Autodesk Inventor part; units mm, degrees
ref_plane "YZ Plane" through (0, 0, 0) normal (1, 0, 0) x (0, 1, 0)
ref_plane "XZ Plane" through (0, 0, 0) normal (0, 1, 0) x (-1, 0, 0)
ref_plane "XY Plane" through (0, 0, 0) normal (0, 0, 1) x (1, 0, 0)
sketch "Sketch3" plane through (0, 0, 0) normal (0, 1, 0) x (-1, 0, 0)
  line L0 (-11.3909, 27.5) -> (11.3909, 27.5)
  line L1 (11.3909, 27.5) -> (27.5, 11.3909)
  line L2 (27.5, 11.3909) -> (27.5, -11.3909)
  line L3 (27.5, -11.3909) -> (11.3909, -27.5)
  line L4 (11.3909, -27.5) -> (-11.3909, -27.5)
  line L5 (-11.3909, -27.5) -> (-27.5, -11.3909)
  line L6 (-27.5, -11.3909) -> (-27.5, 11.3909)
  line L7 (-27.5, 11.3909) -> (-11.3909, 27.5)
  circle A0 centre (0, 0) radius 29.7658
  circle A1 centre (0, 0) radius 27.5
  circle A2 centre (0, 0) radius 21
  circle A3 centre (0, 0) radius 31.7658
  line L8 (0, 0) -> (-27.5, 0)
  line L9 (-27.5, 0) -> (-27.5, 83)
  line L10 (-27.5, 83) -> (0, 83)
  line L11 (0, 83) -> (0, 0)
  line L12 (0, 83) -> (-7.5939, 83)
  line L13 (-7.5939, 83) -> (-7.5939, 166)
  line L14 (-7.5939, 166) -> (0, 166)
  line L15 (0, 166) -> (0, 83)
  line L16 (0, 166) -> (-47, 166)
  line L17 (-47, 166) -> (-47, 171)
  line L18 (-47, 171) -> (0, 171)
  line L19 (0, 171) -> (0, 166)
  circle A4 centre (-47, 168.5) radius 7.5939
  dimension "oSW" = 55
  dimension "oIntDia" = 42
  dimension "d16" = 2
  dimension "oWheelDia" = 94
  dimension "d51" = 5
  dimension "d52" = 15.1878
  dimension "oStemHeight" = 171
  dimension "d57" = 15.1878
  dimension "d58" = 22.7817
revolve "Revolution1" add sketch "Sketch3" angle 360 about axis through (0, 0, 166) along (0, 0, -1) picked at (-6.365, 27.9172) picked at (-16.0373, 26.4927) picked at (-1.7883, 25.1572) picked at (-13.8245, 1.5576) contours A0 L11 L0 | L0 A1 L7 | L7 A0 | A0 L9 A3 L11 | L11 A2 L8 A1 | A1 L6 L7 | L11 L8 A2 | L9 L10 L11 A3 | L10 L13 L14 L15 | L14 L16 A4 L18 L19 | A4 L18 L17 L16 | L16 L17 L18 A4
extrude "Extrusion1" add sketch "Sketch3" along normal mid plane 82 separate body contours L0 A1 L7 | L0 L1 A1 | L11 A2 L8 A1 | A1 L8 A2 L11 | A1 L6 L7 | L1 L2 A1 | A1 L5 L6 | L2 L3 A1 | A1 L4 L5 | L3 L4 A1
extrude "Extrusion12" cut sketch "Sketch3" along normal through all both and the other way through all contours L11 L8 A2 | A2 L8 L11
extrude "Extrusion2" add sketch "Sketch3" along normal mid plane 60 contours A0 L11 L0 | L7 A0 | A0 L9 A3 L11 | L11 A0 L0 | L6 A0 | A0 L11 A3 L9 | A0 L1 | L5 A0 | A0 L2 | L4 A0 | A0 L3
sketch "Sketch10" plane through (0, 41, 0) normal (0, 1, 0) x (1, 0, 0)
  circle A0 centre (0, 0) radius 21
  circle A1 centre (0, 0) radius 21.25
  dimension "d44" = 0.25
extrude "Extrusion11" cut sketch "Sketch10" against normal blind 12
mirror "Mirror1" about plane through (0, 0, 0) normal (0, 1, 0) of "Extrusion11"
equation "\"d52\" = 0.666667 * d58"
equation "\"d57\" = d52"
properties part number "Manual Threaded Ball Valve DN40 S235" material "S235"
Here's how the part is built. I have some questions about the finished solid (model axes, mm). A direction names the side the tool comes from. Give positions to 0.01 mm unless a question says otherwise; leave off trailing zeros. Order: outer loops, then holes, each group sorted by start corner. A loop starts at its lowest first (then second) coordinate and runs counter-clockwise, first axis right, second up. Notation, with made-up numbers: M -12.75,57 L 20.25,57 A34 ccw 20.25,95 Z; hole C 46.25,-18 d6. An arc over 180 degrees is marked long. Use a Markdown table: item, result. Add a question column.
1. For pin 1 Ø9 at (y, z) = (-35, 1.5) entering from +X; pin 2 Ø10 at (x, y) = (-33, 5) entering from +Z; pin 3 Ø10 at (x, z) = (25, 80.5) entering from -Y, each with a flat end and sliding along its axis, tell me the tip position at first contact or that it passes through.
2. I need wall thicknesses on probe 1 along Z at (x, y) = (0, -32.25); probe 2 along X at (y, z) = (14, 0); probe 3 along X at (y, z) = (-33, 0). Which ranges of each line are inside material? Lowest first, please. Write a range as from..to.
3. If we mould it in two halves opening along Z, with no side actions, what happens to faces 4 (the flat face through (-1, -1, 171)), 5 (the cylindrical face through (-16.863, -35.084, -12.93)), 6 (the flat face through (27.5, 35, 0)), 7 (the flat face through (19.33, -35.58, -19.56))? For each: +Z half, -Z half, draft (parallel to the pull), parting line (faces both ways), or undercut.
4. On a 3-axis mill with a long thin cutter (end or side, diameter ignored), from which of +Z, -Z, +X, -X, +Y, -Y can I reach the whole of each face in a straight line? I mean faces 1 (the flat face through (-19.33, -35.58, 19.56)), 2 (the flat face through (-1, 8, 166)), 3 (the flat face through (19.56, -35.58, 19.33)). Say none if no direction works.
5. Suppose I cut it at B-B (y = 0). List the corners of the cut face in (x, z) for me.
6. Suppose I cut it at D-D (z = 92.5). List the corners of the cut face in (x, y) for me.
7. Suppose I cut it at C-C (y = -25). Give the number of separate pieces and of enclosed holes in the cut face, and give its area (3 significant figures).
8. Suppose I cut it at A-A (z = 0). List the corners of the cut face in (x, y) for me, and give its area (3 significant figures).
Results list:
| question | item | result |
|---|---|---|
| 1 | pin 1 | stops at x = 27.5 |
| 1 | pin 2 | stops at z = 171 |
| 1 | pin 3 | stops at y = -18.87 |
| 2 | probe 1 | z = -27.5..-21.25, 21.25..27.5, 166..171 |
| 2 | probe 2 | x = -31.77..-21, 21..31.77 |
| 2 | probe 3 | x = -27.5..-21.25, 21.25..27.5 |
| 3 | face 4 | +Z half |
| 3 | face 5 | undercut |
| 3 | face 6 | draft |
| 3 | face 7 | -Z half |
| 4 | face 1 | -X, -Y |
| 4 | face 2 | none |
| 4 | face 3 | +X, -Y |
| 5 | outline | M -39.83,166 L -7.59,166 L -7.59,83 L -27.5,83 L -27.5,15.9 A31.77 ccw long 27.5,15.9 L 27.5,83 L 7.59,83 L 7.59,166 L 39.83,166 A7.59 ccw long 39.83,171 L -39.83,171 A7.59 ccw long Z; hole C 0,0 d42 |
| 6 | outline | C 0,0 d15.19 |
| 7 | separate pieces | 2 |
| 7 | enclosed holes | 1 |
| 7 | area | 3,710 mm² |
| 8 | outline | M -31.77,-30 L -27.5,-30 L -27.5,-41 L -21.25,-41 L -21.25,-29 L -21,-29 L -21,29 L -21.25,29 L -21.25,41 L -27.5,41 L -27.5,30 L -31.77,30 Z; M 21,-29 L 21.25,-29 L 21.25,-41 L 27.5,-41 L 27.5,-30 L 31.77,-30 L 31.77,30 L 27.5,30 L 27.5,41 L 21.25,41 L 21.25,29 L 21,29 Z |
| 8 | area | 1,570 mm² |
